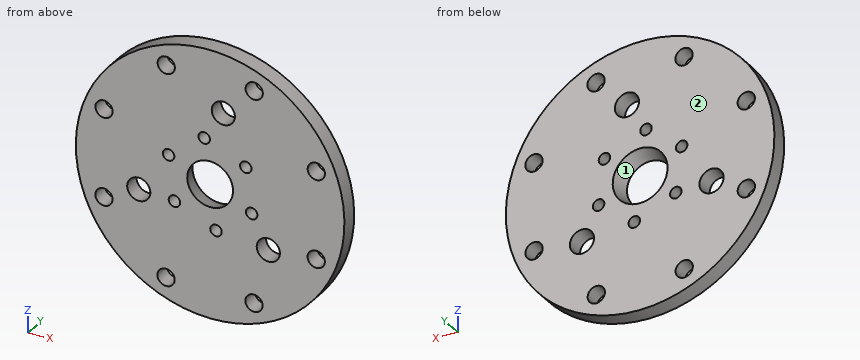
```python
from build123d import *

# Parameters (mm, degrees)
SKETCH1_R               = 76.2
BOSS_EXTRUDE1_DEPTH     = 9.525
CIRPATTERN6_COUNT       = 3
F_3_8_CLEARANCE_HOLE1_D = 9.8044
F_1_4_CLEARANCE_HOLE1_D = 6.5278


with BuildPart() as part:
    # Sketch1 → Boss-Extrude1 (new body)
    with BuildSketch(Plane(origin=(0, 0, 0), x_dir=(1, 0, 0), z_dir=(0, 1, 0))):
        with Locations(Location((0, 0, 0), (0, 0, 90))):
            Circle(SKETCH1_R)
    extrude(amount=BOSS_EXTRUDE1_DEPTH)

    # Sketch5 → Cut-Revolve1 (revolve, cut)
    with BuildSketch(Plane.XY, mode=Mode.PRIVATE) as cut_revolve1_sk:
        Polygon((0, 0), (0, 9.525), (15.552216058, 9.525), (13, 0), align=None)
    revolve(cut_revolve1_sk.sketch.rotate(Axis((0, 0, 0), (0, 1, 0)), 90), axis=Axis((0, 0, 0), (0, 1, 0)), mode=Mode.SUBTRACT)

    # Sketch15 → 1/4 NPT Tapped Hole1 (revolve, cut)
    with BuildSketch(Plane(origin=(33.011727721, 9.525, -27.700128555), x_dir=(0, 0, 1), z_dir=(1, 0, 0))):
        Polygon((0, 0), (0, 9.525), (5.5626, 9.525), (5.5626, 10.0203), (6.557978799, 10.0203), (6.858, 0), align=None)
    f_1_4_npt_tapped_hole1 = revolve(axis=Axis((33.011727721, 15.875, -27.700128555), (0, -1, 0)), mode=Mode.SUBTRACT)

    # CirPattern6: 1/4 NPT Tapped Hole1 ×3 about axis
    cirpattern6_axis = Axis((0, 0, 0), (0, 1, 0))
    for i in range(1, CIRPATTERN6_COUNT):
        add(f_1_4_npt_tapped_hole1.rotate(cirpattern6_axis, i * 360 / CIRPATTERN6_COUNT), mode=Mode.SUBTRACT)

    # 3/8 Clearance Hole1 (through all)
    with Locations(Plane(origin=(0, 9.525, 0), x_dir=(1, 0, 0), z_dir=(0, 1, 0))):
        with Locations((60.207217661, 25.013604371), (60.257374801, -24.888494705), (24.885638551, 60.264250563), (-25.016460514, 60.214093421), (-60.267106699, 24.892514335), (-60.216949569, -25.009584719), (-24.895370482, -60.260230921), (25.006728592, -60.210073801)):
            Hole(F_3_8_CLEARANCE_HOLE1_D / 2)

    # 1/4 Clearance Hole1 (through all)
    with Locations(Plane(origin=(0, 9.525, 0), x_dir=(1, 0, 0), z_dir=(0, 1, 0))):
        with Locations((3.330049479, 25.294237026), (-20.240427094, 15.531025958), (20.240427094, -15.531025958), (-23.570476573, -9.763211068), (-3.330049479, -25.294237026), (23.570476573, 9.763211068)):
            Hole(F_1_4_CLEARANCE_HOLE1_D / 2)


solid = part.part
```
The listing builds one solid part. Answer for the finished solid, in the listing's coordinates (mm). Face numbers are marked on the shaded views. Coordinates: 2 decimals unless noted, no trailing zeros. Write each loop counter-clockwise with the first axis right and the second up, starting at its lowest first coordinate (ties: lowest second). Pieces come first, ordered by that corner, then holes. Notation, with made-up numbers: M 88.25,9 L 120.25,9 A9 cw 120.25,13 Z; hole C 60,61 d10. An arc over 180 degrees is marked long. Use a Markdown table: item, result. Add a question column.
1. Section A-A (z = 0) is taken. Give the vertices of the cut face in (x, y) (3 decimals).
2. Section B-B (y = 4) is taken. Count the separate pieces of the cut face and the enclosed holes in it, plus the area to 3 significant figures.
3. Straight lines are drawn through the part: line 1 along X through (y, z) = (0.75, -25.5); line 2 along X through (y, z) = (5.25, -25.5); line 3 along X through (y, z) = (5.5, 24). For each, find the intervals that lie inside material, in ascending order. Write a range as [from, to].
4. For a pull along Z with two mould halves and no side action, classify the marked faces 1 and 2 as +Z half, -Z half, draft (parallel to the pull), parting line (faces both ways), or undercut.
5. Given P1, Ø5, axis at x = 23.57, z = -9.76, coming from the -Y side; P2, Ø3, axis at y = 7, z = 32, coming from the +X side; P3, Ø1.5, axis at y = 7, z = -44.5, coming from the +X side; P4, Ø1, axis at y = 5, z = 47, coming from the -X side, each flat-ended and moving along its own axis, determine where each tip first touches the part or whether it passes through.
Data:
| question | item | result |
|---|---|---|
| 1 | outline | M -76.2,0 L -13,0 L -15.552,9.525 L -76.2,9.525 Z; M 13,0 L 76.2,0 L 76.2,9.525 L 15.552,9.525 Z |
| 2 | separate pieces | 1 |
| 2 | enclosed holes | 18 |
| 2 | area | 16,400 mm2 |
| 3 | line 1 | x = [-71.81, -65.13], [-55.4, 0.07], [6.59, 26.79], [39.23, 55.33], [65.09, 71.81] |
| 3 | line 2 | x = [-71.81, -65.13], [-55.4, 0.07], [6.59, 26.65], [39.37, 55.33], [65.09, 71.81] |
| 3 | line 3 | x = [-72.32, -65.01], [-55.42, -6.33], [-0.33, 55.44], [65.08, 72.32] |
| 4 | face 1 | undercut |
| 4 | face 2 | draft |
| 5 | P1 | passes through |
| 5 | P2 | stops at x = 69.83 |
| 5 | P3 | stops at x = 62.39 |
| 5 | P4 | stops at x = -60.37 |
